Geometry check sheet. Reference: drawing and pictorial views, mm from the part's lowest x, y, z. A direction names the side the tool comes from. Coordinates: 2 decimals unless noted, no trailing zeros. Write each loop counter-clockwise with the first axis right and the second up, starting at its lowest first coordinate (ties: lowest second). Pieces come first, ordered by that corner, then holes. Notation, with made-up numbers: (61, 50) -> (109, 50) arc R29 cw to (109, 84) -> close; hole circle Ø11 at (7.25, 38.25). An arc over 180 degrees is marked (long way). Use a Markdown table: item, result.
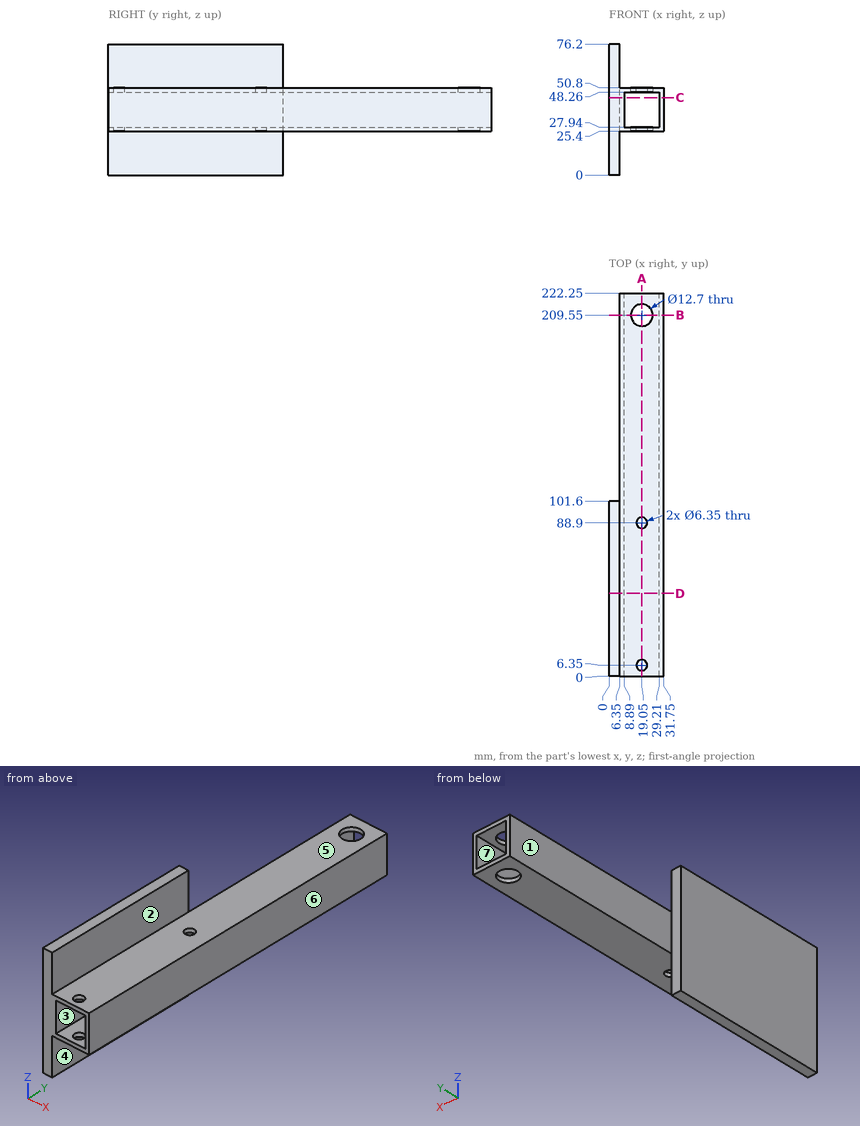
Item 1: Section check A-A on x = 19.05. Count the separate pieces of the cut face and the enclosed holes in it, then the cut area to 4 significant figures.
Answer block:
| item | result |
|---|---|
| separate pieces | 8 |
| enclosed holes | 0 |
| area | 1,000 mm^2 |
Item 2: Depth check by flat-ended pin: P1, Ø16.5, axis at x = 20, y = 127, coming from the +Z side; P2, Ø12.5, axis at y = 44, z = 67, coming from the +X side; P3, Ø10, axis at x = 14.5, y = 92, coming from the -Z side. Enter the tip coordinate at first touch or a pass-through.
Answer block:
| item | result |
|---|---|
| P1 | stops at z = 50.8 |
| P2 | stops at x = 6.35 |
| P3 | stops at z = 25.4 |
Item 3: Thickness scan on L1, parallel to Y at x = 19.05, z = 26.8 (3 decimals); L2, parallel to Z at x = 9.5, y = 189; L3, parallel to X at y = 113, z = 43. Record the ranges inside material, lowest first. Write a range as [from, to].
Answer block:
| item | result |
|---|---|
| L1 | y = [0, 3.175], [9.525, 85.725], [92.075, 203.2], [215.9, 222.25] |
| L2 | z = [25.4, 27.94], [48.26, 50.8] |
| L3 | x = [6.35, 8.89], [29.21, 31.75] |
Item 4: Section check B-B on y = 209.55. Record the boundary of the cut face in (x, z).
Answer block:
| item | result |
|---|---|
| outline | (6.35, 25.4) -> (12.7, 25.4) -> (12.7, 27.94) -> (8.89, 27.94) -> (8.89, 48.26) -> (12.7, 48.26) -> (12.7, 50.8) -> (6.35, 50.8) -> close; (25.4, 25.4) -> (31.75, 25.4) -> (31.75, 50.8) -> (25.4, 50.8) -> (25.4, 48.26) -> (29.21, 48.26) -> (29.21, 27.94) -> (25.4, 27.94) -> close |
Item 5: Section check D-D on y = 48. Record the boundary of the cut face in (x, z).
Answer block:
| item | result |
|---|---|
| outline | (0, 0) -> (6.35, 0) -> (6.35, 25.4) -> (31.75, 25.4) -> (31.75, 50.8) -> (6.35, 50.8) -> (6.35, 76.2) -> (0, 76.2) -> close; hole (8.89, 27.94) -> (29.21, 27.94) -> (29.21, 48.26) -> (8.89, 48.26) -> close |
Item 6: Mould release check, pull along Z, two halves, no side actions. Record for the marked faces 5, 6 and 7: +Z half, -Z half, draft (parallel to the pull), parting line (faces both ways), or undercut.
Answer block:
| item | result |
|---|---|
| face 5 | +Z half |
| face 6 | draft |
| face 7 | undercut |
Item 7: Tool access check on the marked faces 1, 2, 3 and 4. Record the directions out of +Z, -Z, +X, -X, +Y, -Y that give a thin tool (end or side, any length) a straight path to the whole face; none if there is none.
Answer block:
| item | result |
|---|---|
| face 1 | +Z, -Z, -X, +Y |
| face 2 | +Z, +X, +Y, -Y |
| face 3 | +Y, -Y |
| face 4 | -Z, +X, +Y, -Y |
Item 8: Section check C-C on z = 45. Record the boundary of the cut face in (x, y).
Answer block:
| item | result |
|---|---|
| outline | (0, 0) -> (8.89, 0) -> (8.89, 222.25) -> (6.35, 222.25) -> (6.35, 101.6) -> (0, 101.6) -> close; (29.21, 0) -> (31.75, 0) -> (31.75, 222.25) -> (29.21, 222.25) -> close |
